The drawing under review shows one solid part. Ordinate dimensions are in mm from its lowest x, y, z. A direction names the side the tool comes from. Round coordinates to 2 decimals unless told otherwise and drop trailing zeros. Order: outer loops, then holes, each group sorted by start corner. A loop starts at its lowest first (then second) coordinate and runs counter-clockwise, first axis right, second up. Notation, with made-up numbers: (-1.75, 78.5) - (9.25, 78.5) arc R23 ccw to (9.25, 97.5) - close; hole circle Ø2 at (84, -1). An arc over 180 degrees is marked (long way). Answer as a JSON object with one key per item and string values. Group by question number.
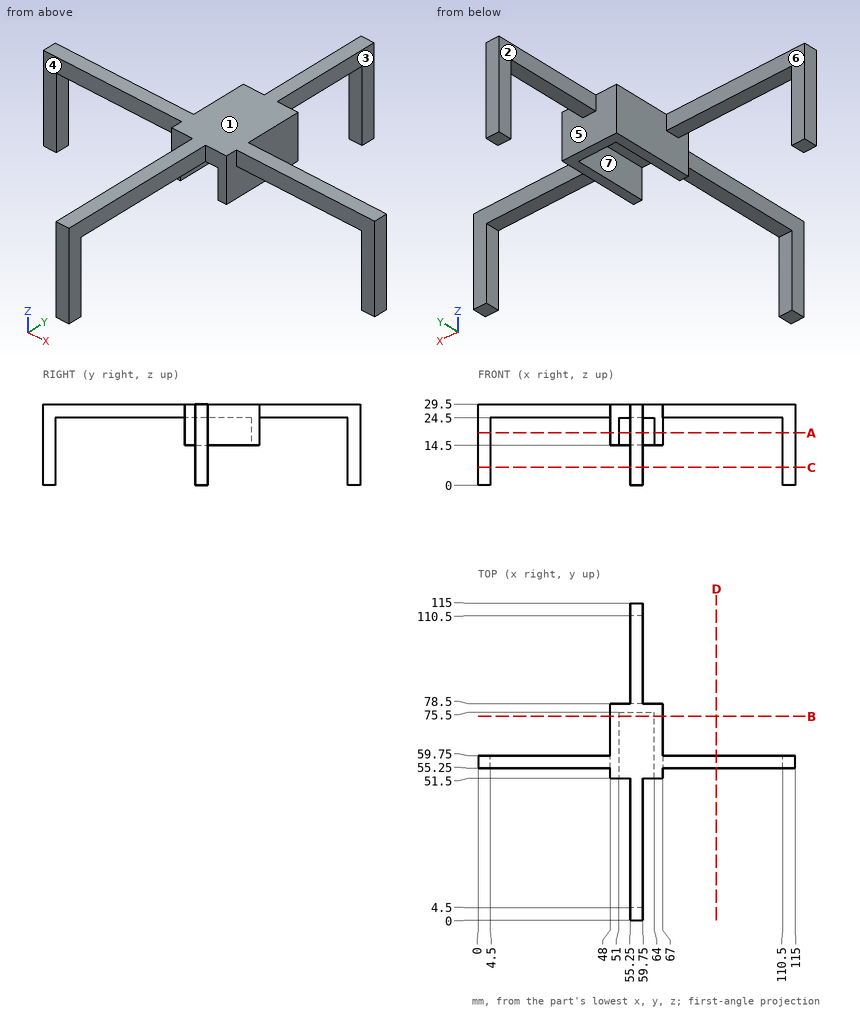
1. Take a section at D-D, the plane x = 86.5. Give the boundary of the cut face in (y, z), then the cut area to 3 significant figures.
2. To check wall thickness, follow line 1 (X direction, y = 55, z = 19.5); line 2 (X direction, y = 73, z = 27.25); line 3 (Y direction, x = 108, z = 25). State the ranges of each line that lie inside material, in increasing order. Write a range as from..to.
3. Take a section at B-B, the plane y = 74. Give the boundary of the cut face in (x, z), then the cut area to 3 significant figures.
4. Mouldability with a two-part tool opening along Y and no side actions: class the marked faces 4, 5, 6 and 7 as pulls with the +Y half, pulls with the -Y half, needs draft (parallel to the pull), parting line crosses it, or undercut.
5. Tool access review of the marked faces 1, 2 and 3: name each direction out of +Z, -Z, +X, -X, +Y, -Y from which nothing blocks a thin tool from reaching the whole face with its end or side.
6. Clearance check with flat-ended pins moving along their axes: P1, Ø12, axis at y = 58, z = 26.5, coming from the -X side; P2, Ø2, axis at x = 57, y = 91.5, coming from the -Z side; P3, Ø3.5, axis at x = 65, z = 25.5, coming from the -Y side; P4, Ø15, axis at y = 98, z = 21.5, coming from the +X side. State where each tip first meets the part, or that it passes through.
7. Take a section at A-A, the plane z = 19. Give the boundary of the cut face in (x, y).
8. Take a section at C-C, the plane z = 6.5. Give the boundary of the cut face in (x, y), then the cut area to 3 significant figures.
Response values:
{
 "1": {"outline": "(55.25, 24.5) - (59.75, 24.5) - (59.75, 29.5) - (55.25, 29.5) - close", "area": "22.5 mm2"},
 "2": {"line 1": "48..51, 64..67", "line 2": "48..67", "line 3": "55.25..59.75"},
 "3": {"outline": "(48, 14.5) - (51, 14.5) - (51, 24.5) - (64, 24.5) - (64, 14.5) - (67, 14.5) - (67, 29.5) - (48, 29.5) - close", "area": "155 mm2"},
 "4": {"face 4": "pulls with the -Y half", "face 5": "undercut", "face 6": "pulls with the +Y half", "face 7": "needs draft"},
 "5": {"face 1": "+Z, +X, -X, +Y, -Y", "face 2": "+Z, -Z, -X, +Y", "face 3": "+Z, -Z, +X, +Y"},
 "6": {"P1": "x = 0", "P2": "z = 24.5", "P3": "y = 51.5", "P4": "x = 59.75"},
 "7": {"outline": "(0, 55.25) - (4.5, 55.25) - (4.5, 59.75) - (0, 59.75) - close; (48, 51.5) - (51, 51.5) - (51, 75.5) - (64, 75.5) - (64, 51.5) - (67, 51.5) - (67, 78.5) - (48, 78.5) - close; (55.25, 0) - (59.75, 0) - (59.75, 4.5) - (55.25, 4.5) - close; (55.25, 110.5) - (59.75, 110.5) - (59.75, 115) - (55.25, 115) - close; (110.5, 55.25) - (115, 55.25) - (115, 59.75) - (110.5, 59.75) - close"},
 "8": {"outline": "(0, 55.25) - (4.5, 55.25) - (4.5, 59.75) - (0, 59.75) - close; (55.25, 0) - (59.75, 0) - (59.75, 4.5) - (55.25, 4.5) - close; (55.25, 110.5) - (59.75, 110.5) - (59.75, 115) - (55.25, 115) - close; (110.5, 55.25) - (115, 55.25) - (115, 59.75) - (110.5, 59.75) - close", "area": "81.0 mm2"}
}
